Design review of the part built by this model. Coordinates are the model's own, in mm. A direction names the side the tool comes from. Coordinates: 2 decimals unless noted, no trailing zeros. Loops run counter-clockwise (first coordinate to the right, second up) from the corner with the lowest first, then second, coordinate; pieces in that order, holes last. Notation, with made-up numbers: (-3.75, 56) -> (10.25, 56) arc R11 ccw to (10.25, 66) -> close; hole circle Ø9 at (-36, -3.5). An arc over 180 degrees is marked (long way). Use a Markdown table: item, result. Add a question column.
Q1. Draft analysis for pull direction X (two halves, no side actions). For faces 5 (the face through (-4465.053, 49, 2448)), 6 (the face through (-4366, 10, 2376)), 7 (the face through (-4366, 0, 2445)), state which applies: pulls with the +X half, pulls with the -X half, needs draft (parallel to the pull), parting line crosses it, or undercut.
Q2. Take a section at D-D on y = 39. Write out the cut boundary in (x, z), plus the area to 3 significant figures.
Q3. Take a section at C-C on x = -4378. Write out the cut boundary in (y, z).
Q4. For faces 1 (the face through (-4366, 38, 2346.684)), 2 (the face through (-4287.55, 20.11, 2541.75)), 3 (the face through (-4369.822, 51.502, 2351.614)), 4 (the face through (-4430, 10, 2468)), list the 3-axis set-ups (+Z, -Z, +X, -X, +Y, -Y) from which the entire face can be reached by the end or side of a thin tool; tool diameter is ignored.
Q5. Clearance check with flat-ended pins moving along their axes: pin 1 Ø4 at (x, y) = (-4285.05, 20) entering from +Z; pin 2 Ø2 at (x, z) = (-4337, 2387) entering from -Y; pin 3 Ø3 at (x, z) = (-4391, 2508.5) entering from +Y. State where each tip first meets the part, or that it passes through.
Q6. Take a section at B-B on z = 2415. Write out the cut boundary in (x, y), plus the area to 3 significant figures.
Q7. Take a section at A-A on y = 14. Write out the cut boundary in (x, z).
Q8. For probe 1 along Z at (x, y) = (-4453, 24); probe 2 along X at (y, z) = (12, 2404); probe 3 along Z at (x, y) = (-4369, 39.5), list the stretches that pass through material, from the lowest coordinate up.
from build123d import *

# Parameters (mm, degrees)
SKETCH1_W           = 200
SKETCH1_H           = 200
SKETCH1_W_2         = 180
SKETCH1_H_2         = 180
BOSS_EXTRUDE1_DEPTH = 100
SKETCH2_W           = 200
SKETCH2_H           = 200
BOSS_EXTRUDE2_DEPTH = 10
SKETCH3_R           = 5
CUT_EXTRUDE1_DEPTH  = 10
SKETCH4_W           = 5
SKETCH4_H           = 135
BOSS_EXTRUDE3_DEPTH = 20
SKETCH6_R           = 2.5
CUT_EXTRUDE2_DEPTH  = 10


with BuildPart() as part:
    # Sketch1 → Boss-Extrude1 (new body)
    with BuildSketch(Plane(origin=(0, 0, 0), x_dir=(1, 0, 0), z_dir=(0, 1, 0))):
        with Locations((-4365.052631579, -2446.684210526)):
            Rectangle(SKETCH1_W, SKETCH1_H)
        with Locations((-4365.052631579, -2446.684210526)):
            Rectangle(SKETCH1_W_2, SKETCH1_H_2, mode=Mode.SUBTRACT)
    extrude(amount=BOSS_EXTRUDE1_DEPTH)

    # Sketch2 → Boss-Extrude2 (add)
    with BuildSketch(Plane(origin=(0, 0, 0), x_dir=(1, 0, 0), z_dir=(0, 1, 0))):
        with Locations((-4365.052631579, -2446.684210526)):
            Rectangle(SKETCH2_W, SKETCH2_H)
    extrude(amount=BOSS_EXTRUDE2_DEPTH)

    # Sketch3 → Cut-Extrude1 (cut)
    with BuildSketch(Plane(origin=(0, 0, 2346.684210526), x_dir=(-1, 0, 0), z_dir=(0, 0, -1))):
        with Locations((4365.052631579, 50)):
            Circle(SKETCH3_R)
    extrude(amount=-CUT_EXTRUDE1_DEPTH, mode=Mode.SUBTRACT)

    # Sketch4 → Boss-Extrude3 (add)
    with BuildSketch(Plane(origin=(0, 10, 0), x_dir=(1, 0, 0), z_dir=(0, 1, 0))):
        with Locations((-4402.552631579, -2469.184210526)):
            Rectangle(SKETCH4_W, SKETCH4_H)
        Polygon((-4275.052631579, -2396.684210526), (-4455.052631579, -2396.684210526), (-4455.052631579, -2401.684210526), (-4405.052631579, -2401.684210526), (-4400.052631579, -2401.684210526), (-4275.052631579, -2401.684210526), align=None)
    extrude(amount=BOSS_EXTRUDE3_DEPTH)

    # Sketch6 → Cut-Extrude2 (cut)
    with BuildSketch(Plane.XY.offset(2546.684210526)):
        with Locations((-4285.052631579, 20)):
            Circle(SKETCH6_R)
    extrude(amount=-CUT_EXTRUDE2_DEPTH, mode=Mode.SUBTRACT)


solid = part.part
Answer list:
| question | item | result |
|---|---|---|
| 1 | face 5 | pulls with the -X half |
| 1 | face 6 | undercut |
| 1 | face 7 | needs draft |
| 2 | outline | (-4465.05, 2346.68) -> (-4265.05, 2346.68) -> (-4265.05, 2546.68) -> (-4465.05, 2546.68) -> close; hole (-4455.05, 2356.68) -> (-4275.05, 2356.68) -> (-4275.05, 2536.68) -> (-4455.05, 2536.68) -> close |
| 2 | area | 7,600 mm² |
| 3 | outline | (0, 2346.68) -> (100, 2346.68) -> (100, 2356.68) -> (10, 2356.68) -> (10, 2396.68) -> (30, 2396.68) -> (30, 2401.68) -> (10, 2401.68) -> (10, 2536.68) -> (100, 2536.68) -> (100, 2546.68) -> (0, 2546.68) -> close |
| 4 | face 1 | -Z, +X, -X, +Y, -Y |
| 4 | face 2 | +Z |
| 4 | face 3 | -Z |
| 4 | face 4 | +Y |
| 5 | pin 1 | z = 2401.68 |
| 5 | pin 2 | y = 0 |
| 5 | pin 3 | y = 10 |
| 6 | outline | (-4465.05, 0) -> (-4265.05, 0) -> (-4265.05, 100) -> (-4275.05, 100) -> (-4275.05, 10) -> (-4400.05, 10) -> (-4400.05, 30) -> (-4405.05, 30) -> (-4405.05, 10) -> (-4455.05, 10) -> (-4455.05, 100) -> (-4465.05, 100) -> close |
| 6 | area | 3,900 mm² |
| 7 | outline | (-4465.05, 2346.68) -> (-4265.05, 2346.68) -> (-4265.05, 2546.68) -> (-4465.05, 2546.68) -> close; hole (-4455.05, 2356.68) -> (-4275.05, 2356.68) -> (-4275.05, 2396.68) -> (-4455.05, 2396.68) -> close; hole (-4455.05, 2401.68) -> (-4405.05, 2401.68) -> (-4405.05, 2536.68) -> (-4455.05, 2536.68) -> close; hole (-4400.05, 2401.68) -> (-4275.05, 2401.68) -> (-4275.05, 2536.68) -> (-4400.05, 2536.68) -> close |
| 8 | probe 1 | 2346.68 to 2356.68, 2396.68 to 2401.68, 2536.68 to 2546.68 |
| 8 | probe 2 | -4465.05 to -4455.05, -4405.05 to -4400.05, -4275.05 to -4265.05 |
| 8 | probe 3 | 2346.68 to 2356.68, 2536.68 to 2546.68 |
